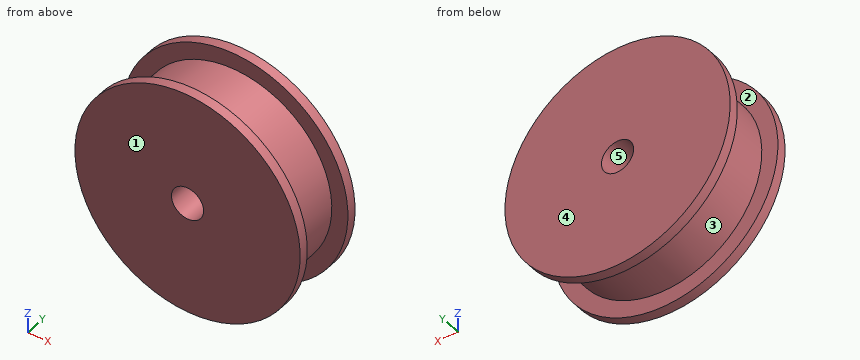
from build123d import *

# Parameters (mm, degrees)
SKETCH_205_R        = 15
EXTRUDE_1_DEPTH     = 5
EXTRUDE_START       = 5
SKETCH_286_R        = 17.5
EXTRUDE_1_2_DEPTH   = 1.5
EXTRUDE_START_2     = -5
SKETCH_2_2_R        = 17.5
EXTRUDE_2_DEPTH     = 1.5
SKETCH_407_R        = 2.5
CUT_EXTRUDE_1_DEPTH = 6.5


with BuildPart() as part:
    # Sketch 205 → Extrude 1 (new, symmetric)
    with BuildSketch(Plane(origin=(0, 0, 0), x_dir=(1, 0, 0), z_dir=(0, 1, 0))):
        with Locations(Location((0, 0, 0), (0, 0, 270))):
            Circle(SKETCH_205_R)
    extrude(amount=EXTRUDE_1_DEPTH, both=True)

    # Sketch 286 → Extrude 1 2 (add)
    with BuildSketch(Plane(origin=(0, 0, 0), x_dir=(1, 0, 0), z_dir=(0, 1, 0)).offset(EXTRUDE_START)):
        with Locations(Location((0, 0, 0), (0, 0, 270))):
            Circle(SKETCH_286_R)
    extrude(amount=EXTRUDE_1_2_DEPTH)

    # 草图2<2> → 边缘2 (add)
    with BuildSketch(Plane(origin=(0, 0, 0), x_dir=(1, 0, 0), z_dir=(0, 1, 0)).offset(EXTRUDE_START_2)):
        with Locations(Location((0, 0, 0), (0, 0, 270))):
            Circle(SKETCH_2_2_R)
    extrude(amount=EXTRUDE_2_DEPTH)

    # Sketch 407 → 切除-拉伸1 (cut, symmetric)
    with BuildSketch(Plane(origin=(0, 0, 0), x_dir=(1, 0, 0), z_dir=(0, 1, 0))):
        with Locations(Location((0, 0, 0), (0, 0, 270))):
            Circle(SKETCH_407_R)
    extrude(amount=CUT_EXTRUDE_1_DEPTH, both=True, mode=Mode.SUBTRACT)


solid = part.part
Design review of the part built by this model. Coordinates are the model's own, in mm. Face numbers are marked on the shaded views. A direction names the side the tool comes from. Give positions to 0.01 mm unless a question says otherwise; leave off trailing zeros. Write each loop counter-clockwise with the first axis right and the second up, starting at its lowest first coordinate (ties: lowest second). Pieces come first, ordered by that corner, then holes. Notation, with made-up numbers: M 23.25,42.25 L 42.25,42.25 A25 ccw 42.25,57.25 Z; hole C 57,89.5 d7. An arc over 180 degrees is marked long. Answer as a JSON object with one key per item and string values. Group by question number.
1) Tool access review of the marked faces 1 and 2: name each direction out of +Z, -Z, +X, -X, +Y, -Y from which nothing blocks a thin tool from reaching the whole face with its end or side.
2) Clearance check with flat-ended pins moving along their axes: pin 1 Ø2 at (x, y) = (0, 3) entering from -Z; pin 2 Ø2 at (y, z) = (-0.5, 7) entering from -X; pin 3 Ø4.5 at (x, z) = (0, 0) entering from -Y. State where each tip first meets the part, or that it passes through.
3) We need section D-D (z = -10). Give the boundary of the cut face in (x, y), and give its area (3 significant figures).
4) For line 1 along X through (y, z) = (5.25, 0); line 2 along Y through (x, z) = (12, 10.5); line 3 along X through (y, z) = (-1, 0), list the stretches that pass through material, from the lowest coordinate up.
5) We need section A-A (x = 0). Give the boundary of the cut face in (y, z).
6) Mouldability with a two-part tool opening along X and no side actions: class the marked faces 3, 4 and 5 as released by +X, released by -X, zero draft, split by the parting line, or undercut.
7) We need section C-C (y = 1.25). Give the boundary of the cut face in (x, z), and give its area (3 significant figures).
8) We need section B-B (z = 0). Give the boundary of the cut face in (x, y), and give its area (4 significant figures).
Answer key:
{
 "1": {"face 1": "+Z, -Z, +X, -X, -Y", "face 2": "none"},
 "2": {"pin 1": "stops at z = -15", "pin 2": "stops at x = -13.75", "pin 3": "passes through"},
 "3": {"outline": "M -14.36,-5 L 14.36,-5 L 14.36,-3.5 L 11.18,-3.5 L 11.18,5 L 14.36,5 L 14.36,6.5 L -14.36,6.5 L -14.36,5 L -11.18,5 L -11.18,-3.5 L -14.36,-3.5 Z", "area": "276 mm²"},
 "4": {"line 1": "x = -17.5 to -2.5, 2.5 to 17.5", "line 2": "y = -5 to -3.5, 5 to 6.5", "line 3": "x = -15 to -2.5, 2.5 to 15"},
 "5": {"outline": "M -5,-17.5 L -3.5,-17.5 L -3.5,-15 L 5,-15 L 5,-17.5 L 6.5,-17.5 L 6.5,-2.5 L -5,-2.5 Z; M -5,2.5 L 6.5,2.5 L 6.5,17.5 L 5,17.5 L 5,15 L -3.5,15 L -3.5,17.5 L -5,17.5 Z"},
 "6": {"face 3": "split by the parting line", "face 4": "zero draft", "face 5": "undercut"},
 "7": {"outline": "C 0,0 d30; hole C 0,0 d5", "area": "687 mm²"},
 "8": {"outline": "M -17.5,-5 L -2.5,-5 L -2.5,6.5 L -17.5,6.5 L -17.5,5 L -15,5 L -15,-3.5 L -17.5,-3.5 Z; M 2.5,-5 L 17.5,-5 L 17.5,-3.5 L 15,-3.5 L 15,5 L 17.5,5 L 17.5,6.5 L 2.5,6.5 Z", "area": "302.5 mm²"}
}
